Geometry check sheet. Reference: the model listing, model coordinates, mm. A direction names the side the tool comes from. Round coordinates to 2 decimals unless told otherwise and drop trailing zeros. Write each loop counter-clockwise with the first axis right and the second up, starting at its lowest first coordinate (ties: lowest second). Pieces come first, ordered by that corner, then holes.
Item 1: Scan lines: probe 1 along Y at (x, z) = (45, -16.45); probe 2 along Y at (x, z) = (4.75, 0); probe 3 along X at (y, z) = (12, -23.5). Record each from-to range of solid material in increasing order.
Item 2: Cross-section at C-C (x = 18). Enter the section's corners in (y, z).
Item 3: Draft check along X on faces 1 (the face through (47, 0, 16)), 2 (the face through (38, 18.7, 20.8)), 3 (the face through (43.5, 0.07, -16.23)), 4 (the face through (44, -16, -6)). Enter one of: pulls with the +X half, pulls with the -X half, needs draft (parallel to the pull), parting line crosses it, or undercut.
Item 4: Depth check by flat-ended pin: P1, Ø10, axis at x = 26.5, y = 16.5, coming from the -Z side; P2, Ø6, axis at x = 23.5, z = 7.5, coming from the +Y side; P3, Ø2, axis at x = 44, y = 16.5, coming from the -Z side. Enter the tip coordinate at first touch or a pass-through.
Item 5: Cross-section at D-D (z = 10.5). Enter the section's corners in (x, y), then the cut area to 3 significant figures.
Item 6: Access from +Z, -Z, +X, -X, +Y, -Y to the whole of each face (thin tool, end or side, straight path). Record for faces 5 (the face through (44, -8.25, 16)), 6 (the face through (43, 0, 15)), 7 (the face through (18.255, 24.397, 12.69)).
Item 7: Cross-section at A-A (x = 45). State how many separate pieces and enclosed holes the cut face has, then the cut area to 4 significant figures.
Item 8: Cross-section at B-B (y = -22.5). Enter the section's corners in (x, z), then the cut area to 3 significant figures.
from build123d import *

# Parameters (mm, degrees)
SKETCH_2_R               = 1.5
CUT_EXTRUDE_1_DEPTH      = 8
SKETCH_3_W               = 2.5
SKETCH_3_H               = 16.5
SKETCH_3_W_2             = 12
SKETCH_3_H_2             = 2.5
EXTRUDE_1_DEPTH          = 6
SKETCH_4_R               = 1.5
CUT_EXTRUDE_2_DEPTH      = 50
PATTERN_CIRCULAR_1_COUNT = 2
PATTERN_CIRCULAR_1_ANGLE = 90


with BuildPart() as part:
    # 草图1 → 旋转1 (revolve)
    with BuildSketch(Plane.XY, mode=Mode.PRIVATE) as revolve_1_sk:
        Polygon((1.5, 16.5), (0, 16.5), (0, 16.4), (-2.2, 16.4), (-2.2, 0), (38, 0), (38, 15), (41, 15), (41, 28.2), (38, 28.2), (38, 27.7), (36, 27.7), (36, 27.5), (1, 27.5), (1, 21.5), (1.5, 21.5), align=None)
    revolve(revolve_1_sk.sketch.rotate(Axis((-20.365384615, 0, 0), (1, 0, 0)), 90), axis=Axis((-20.365384615, 0, 0), (1, 0, 0)))

    # 草图2 → 切除-拉伸1 (cut)
    with BuildSketch(Plane.ZY.offset(-1)):
        with Locations((0, 25)):
            Circle(SKETCH_2_R)
        with Locations((21.650635095, -12.5)):
            Circle(SKETCH_2_R)
        with Locations((-21.650635095, -12.5)):
            Circle(SKETCH_2_R)
    extrude(amount=-CUT_EXTRUDE_1_DEPTH, mode=Mode.SUBTRACT)

    # 草图3 → 凸台-拉伸1 (add)
    with BuildSketch(Plane(origin=(41, 0, 0), x_dir=(0, 0, -1), z_dir=(1, 0, 0))):
        with Locations((16.25, 0)):
            Rectangle(SKETCH_3_W, SKETCH_3_H)
        with Locations((0, 16.25)):
            Rectangle(SKETCH_3_W_2, SKETCH_3_H_2)
        with Locations((-16.25, 0)):
            Rectangle(SKETCH_3_W, SKETCH_3_H)
        with Locations((0, -16.25)):
            Rectangle(SKETCH_3_W_2, SKETCH_3_H_2)
    extrude(amount=EXTRUDE_1_DEPTH)

    # 草图4 → 切除-拉伸2 (cut, symmetric)
    with BuildSketch(Plane.XY):
        with Locations((45, 0)):
            Circle(SKETCH_4_R)
    cut_extrude_2 = extrude(amount=CUT_EXTRUDE_2_DEPTH, both=True, mode=Mode.SUBTRACT)

    # 阵列(圆周)1: 切除-拉伸2 ×2 about axis
    pattern_circular_1_axis = Axis((36, 0, 0), (-1, 0, 0))
    for i in range(1, PATTERN_CIRCULAR_1_COUNT):
        add(cut_extrude_2.rotate(pattern_circular_1_axis, i * PATTERN_CIRCULAR_1_ANGLE / (PATTERN_CIRCULAR_1_COUNT - 1)), mode=Mode.SUBTRACT)


solid = part.part
Resolved:
1. probe 1: y = -8.25 to -1.5, 1.5 to 8.25
1. probe 2: y = -27.5 to 23.5, 26.5 to 27.5
1. probe 3: x = 1 to 41
2. outline: circle Ø55 at (0, 0)
3. face 1: pulls with the +X half
3. face 2: pulls with the -X half
3. face 3: undercut
3. face 4: needs draft
4. P1: stops at z = -24.98
4. P2: stops at y = 27.13
4. P3: stops at z = -6
5. outline: (-2.2, -12.6) - (0, -12.6) - (0, -12.73) - (1.5, -12.73) - (1.5, -18.76) - (1, -18.76) - (1, -25.42) - (36, -25.42) - (36, -25.63) - (38, -25.63) - (38, -26.17) - (41, -26.17) - (41, -10.71) - (38, -10.71) - (38, 10.71) - (41, 10.71) - (41, 26.17) - (38, 26.17) - (38, 25.63) - (36, 25.63) - (36, 25.42) - (1, 25.42) - (1, 18.76) - (1.5, 18.76) - (1.5, 12.73) - (0, 12.73) - (0, 12.6) - (-2.2, 12.6) - close
5. area: 2,050 mm2
6. face 5: +Z, -Z, +X, -Y
6. face 6: +X, +Y, -Y
6. face 7: -X
7. separate pieces: 8
7. enclosed holes: 0
7. area: 112.5 mm2
8. outline: (1, -15.81) - (36, -15.81) - (36, -16.16) - (38, -16.16) - (38, -17) - (41, -17) - (41, 17) - (38, 17) - (38, 16.16) - (36, 16.16) - (36, 15.81) - (1, 15.81) - close
8. area: 1,270 mm2
